Can you work these out from the model? Positions are in its coordinate system, mm. A direction names the side the tool comes from. Give positions to 0.01 mm unless a question says otherwise; leave off trailing zeros. Order: outer loops, then holes, each group sorted by start corner. A loop starts at its lowest first (then second) coordinate and runs counter-clockwise, first axis right, second up. Notation, with made-up numbers: M 19.5,81.5 L 31.5,81.5 A18 cw 31.5,95.5 Z; hole C 85.5,-37.75 d3. An arc over 180 degrees is marked long. Answer as a JSON object with one key per item and string values.
```python
from build123d import *

# Parameters (mm, degrees)
SKETCH1_W           = 42.8625
SKETCH1_H           = 42.8625
BOSS_EXTRUDE1_DEPTH = 45
SKETCH4_R           = 17.5
BOSS_EXTRUDE2_DEPTH = 45
SKETCH5_R           = 4
BOSS_EXTRUDE3_DEPTH = 19
CHAMFER1_SIZE       = 3.175
CHAMFER2_SIZE       = 0.79375


with BuildPart() as part:
    # Sketch1 → Boss-Extrude1 (new body)
    with BuildSketch(Plane(origin=(0, 0, 0), x_dir=(0, 0, -1), z_dir=(1, 0, 0))):
        Rectangle(SKETCH1_W, SKETCH1_H)
    extrude(amount=-BOSS_EXTRUDE1_DEPTH)

    # Sketch4 → Boss-Extrude2 (add)
    with BuildSketch(Plane.ZY.offset(45)):
        with Locations(Location((0, 0, 0), (0, 0, 180))):
            Circle(SKETCH4_R)
    extrude(amount=BOSS_EXTRUDE2_DEPTH)

    # Sketch5 → Boss-Extrude3 (add)
    with BuildSketch(Plane.ZY.offset(90)):
        Circle(SKETCH5_R)
    extrude(amount=BOSS_EXTRUDE3_DEPTH)

    # Chamfer1
    chamfer1_edges = [part.edges().sort_by_distance(p)[0] for p in [
        (-22.5, -21.43125, -21.43125),
        (-22.5, -21.43125, 21.43125),
        (-22.5, 21.43125, 21.43125),
        (-22.5, 21.43125, -21.43125),
    ]]
    chamfer(chamfer1_edges, length=CHAMFER1_SIZE)

    # Chamfer2
    chamfer2_edges = [part.edges().sort_by_distance(p)[0] for p in [
        (-90, 0, 17.5),
    ]]
    chamfer(chamfer2_edges, length=CHAMFER2_SIZE)


solid = part.part
```
1) I want a section at D-D on x = -98.5. Write out the boundary of the cut face in (y, z).
Results found:
{"outline": "C 0,0 d8"}
2) I want a section at A-A on y = 0. Write out the boundary of the cut face in (x, z).
Results found:
{"outline": "M -109,-4 L -90,-4 L -90,-16.71 L -89.21,-17.5 L -45,-17.5 L -45,-21.43 L 0,-21.43 L 0,21.43 L -45,21.43 L -45,17.5 L -89.21,17.5 L -90,16.71 L -90,4 L -109,4 Z"}
3) I'm going to push flat-ended pins straight in: pin 1 Ø13 at (y, z) = (-7, -1.5) entering from -X; pin 2 Ø4 at (x, y) = (-86.5, -15.5) entering from +Z; pin 3 Ø10 at (y, z) = (-13.5, 11.5) entering from -X; pin 4 Ø5 at (x, y) = (-62.5, 6) entering from +Z. Where does each tip first touch, or does it pass through?
Results found:
{"pin 1": "stops at x = -109", "pin 2": "stops at z = 11.14", "pin 3": "stops at x = -90", "pin 4": "stops at z = 17.15"}
4) I want a section at C-C on x = -74. Write out the boundary of the cut face in (y, z), and give its area (3 significant figures).
Results found:
{"outline": "C 0,0 d35", "area": "962 mm²"}
5) I need wall thicknesses on L1, parallel to Z at x = -75.5, y = -0.5; L2, parallel to X at y = 5, z = -10.5; L3, parallel to X at y = -13, z = 12. Which ranges of each line are inside material? Lowest first, please.
Results found:
{"L1": "z = -17.49 to 17.49", "L2": "x = -90 to 0", "L3": "x = -45 to 0"}
6) For faces 1 (the face through (-99.367, -3.905, -0.867)), 2 (the face through (-22.18, 19.87, 19.82)), which set-ups out of +Z, -Z, +X, -X, +Y, -Y let a thin tool reach every point of the face, with its end or its side?
Results found:
{"face 1": "-X", "face 2": "+Z, +X, -X, +Y"}
